```python
from build123d import *

# Parameters (mm, degrees)
BASETOP_FACE_RADIUS = 2.6
BASETOP_HEIGHT      = 0.7
CROSSRECESS_DEPTH   = 0.825
DRAFT9_ANGLE        = -30
FILLET5_R           = 0.3


with BuildPart() as part:
    # Sketch1 → Base (revolve)
    with BuildSketch(Plane.XY):
        Polygon((30, 1.5), (2.737867966, 1.5), (1.467367966, 1.5), (0.367367966, 2.6), (0, 2.6), (0, 0), (30, 0), align=None)
    revolve(axis=Axis((4.515812911, 0, 0), (-1, 0, 0)))

    # BaseTop: a dome of height H over a round flat face of radius A is a cap of a sphere of radius (A * A + H * H) / (2 * H)
    basetop_r = (BASETOP_FACE_RADIUS * BASETOP_FACE_RADIUS + BASETOP_HEIGHT * BASETOP_HEIGHT) / (2 * BASETOP_HEIGHT)
    basetop_base = Plane((0, 0, 0), z_dir=(-1, 0, 0))
    with Locations(basetop_base.offset(BASETOP_HEIGHT - basetop_r)):
        basetop_ball = Sphere(basetop_r, mode=Mode.PRIVATE)
    add(split(basetop_ball, bisect_by=basetop_base, keep=Keep.TOP, mode=Mode.PRIVATE))

    # Sketch6 → CrossRecess (cut)
    with BuildSketch(Plane.ZY.offset(0.7)):
        Polygon((0.34, 0.34), (0.34, 1.7), (-0.34, 1.7), (-0.34, 0.34), (-1.7, 0.34), (-1.7, -0.34), (-0.34, -0.34), (-0.34, -1.7), (0.34, -1.7), (0.34, -0.34), (1.7, -0.34), (1.7, 0.34), align=None)
    extrude(amount=-CROSSRECESS_DEPTH, mode=Mode.SUBTRACT)

    # Draft9
    draft9_faces = [part.faces().sort_by_distance(p)[0] for p in [
        (-0.14204754, 0, -1.7),
        (-0.14204754, -1.7, 0),
        (-0.14204754, 0, 1.7),
        (-0.14204754, 1.7, 0),
    ]]
    draft(draft9_faces, Plane(origin=(-0.7, 0, 0), x_dir=(0, 0, 1), z_dir=(1, 0, 0)), DRAFT9_ANGLE)

    # Fillet5
    fillet5_edges = [part.edges().sort_by_distance(p)[0] for p in [
        (-0.27631446, 0.34, -0.34),
        (-0.27631446, 0.34, 0.34),
        (-0.27631446, -0.34, 0.34),
        (-0.27631446, -0.34, -0.34),
    ]]
    fillet(fillet5_edges, radius=FILLET5_R)


solid = part.part
```
Verification items for the finished model (mm, model axes). Coordinates: 2 decimals unless noted, no trailing zeros. Write each loop counter-clockwise with the first axis right and the second up, starting at its lowest first coordinate (ties: lowest second). Pieces come first, ordered by that corner, then holes. Notation, with made-up numbers: (-30, 29.5) - (24, 29.5) arc R22 ccw to (24, 62.5) - close; hole circle Ø8 at (38.25, -11). An arc over 180 degrees is marked (long way). One line per question, with ' | ' between items. Start each with the question number.
1. Gauge pin test, flat ends, axial feed: P1, Ø0.9, axis at x = 0, y = 1, coming from the +Z side; P2, Ø2, axis at x = 23.5, y = -0.5, coming from the -Z side. Record the tip position at first contact, or that the pin passes through.
2. Section check C-C (x = 16). Enter the section's corners in (y, z).
3. Material ranges on line 1 along X through (y, z) = (-0.25, -0.45) (3 decimals); line 2 along Z through (x, y) = (22.5, 0.05); line 3 along X through (y, z) = (1.35, -1.9), recorded low to high.
4. Section check A-A (z = 0). Enter the section's corners in (x, y) (3 decimals), plus the area to 3 significant figures.
5. Draft check along Y on faces 1 (the flat face through (0.125, 0, 0)), 2 (the cylindrical face through (0.181, -0.338, -2.578)), 3 (the flat face through (30, 0, 0)). Enter one of: released by +Y, released by -Y, zero draft, split by the parting line, or undercut.
Computed values:
1) P1: z = 2.54 | P2: z = -1.5
2) outline: circle Ø3 at (0, 0)
3) line 1: 0.125 to 30 | line 2: -1.5 to 1.5 | line 3: -0.15 to 0.64
4) outline: (-0.459, -1.561) arc R5.179 ccw to (0, -2.6) - (0.367, -2.6) - (1.467, -1.5) - (30, -1.5) - (30, 1.5) - (1.467, 1.5) - (0.367, 2.6) - (0, 2.6) arc R5.179 ccw to (-0.459, 1.561) - (0.125, 1.224) - (0.125, -1.224) - close | area: 92.3 mm²
5) face 1: undercut | face 2: split by the parting line | face 3: zero draft
